CAD build for the part. Positions are in the model's coordinates, mm. A direction names the side the tool comes from. Give positions to 0.01 mm unless a question says otherwise; leave off trailing zeros. Order: outer loops, then holes, each group sorted by start corner. A loop starts at its lowest first (then second) coordinate and runs counter-clockwise, first axis right, second up.
Item 1: Band-saw the part on C-C on x = 0. Give the cut face in (y, z), plus the area to 3 significant figures.
Item 2: Band-saw the part on D-D on z = 9.25. Count the separate pieces of the cut face and the enclosed holes in it, plus the area to 3 significant figures.
Item 3: Band-saw the part on A-A on z = 1.25. Give the cut face in (x, y) (3 decimals), plus the area to 3 significant figures.
Item 4: Band-saw the part on B-B on x = 40. Give the cut face in (y, z), plus the area to 3 significant figures.
Item 5: Which spindle directions (+Z, -Z, +X, -X, +Y, -Y) get a long thin tool onto all of the face, cutting with end or side? Do faces 1 (the flat face through (25, 0, 0)), 2 (the flat face through (37.51, -14.46, 8.03)). Say none if no direction does.
Item 6: Wall check: L1, parallel to Y at x = 40, z = 2.5; L2, parallel to X at y = -1.5, z = 1.25; L3, parallel to Z at x = 6, y = -5. Give the ranges that are in metal, low to high.
Item 7: Two-plate mould, pull along X, no slides. Class faces 3 (the cylindrical face through (57.494, -0.447, 4.93)), 4 (the flat face through (16.612, -12.035, 3.819)), 5 (the flat face through (40, 15.5, 8)): released by +X, released by -X, zero draft, split by the parting line, or undercut.
Item 8: Flat gauge pins, fed straight in: P1, Ø5, axis at x = 28.5, z = 8.5, coming from the +Y side; P2, Ø1.4, axis at y = -12, z = 8, coming from the +X side; P3, Ø1.4, axis at x = 27.5, z = 7.5, coming from the -Y side; P4, Ø5.5, axis at x = 40, y = 0, coming from the -Z side. Where does each tip first touch, or does it go through?
```python
from build123d import *

# Parameters (mm, degrees)
SKETCH1_R           = 17.5
SKETCH1_R_2         = 10
SKETCH1_R_3         = 6
SKETCH1_R_4         = 3.5
SKETCH1_R_5         = 7.5
SKETCH1_R_6         = 5
SKETCH1_R_7         = 2
BOSS_EXTRUDE1_DEPTH = 10
SKETCH4_R           = 2
CUT_EXTRUDE2_DEPTH  = 11
CUT_EXTRUDE3_DEPTH  = 4
SKETCH5_R           = 2
CUT_EXTRUDE4_DEPTH  = 3
SKETCH6_R           = 5
CUT_EXTRUDE5_DEPTH  = 4
SKETCH7_R           = 6.5
CUT_EXTRUDE6_DEPTH  = 5


with BuildPart() as part:
    # Sketch1 → Boss-Extrude1 (new body)
    with BuildSketch(Plane.XY):
        with BuildLine():
            Line((35.625, 16.94430214), (-1.875, 7.261843774))
            ThreePointArc((-1.875, 7.261843774), (4.592793268, 5.929270613), (7.5, 0))
            ThreePointArc((7.5, 0), (4.592793268, -5.929270613), (-1.875, -7.261843774))
            Line((-1.875, -7.261843774), (35.625, -16.94430214))
            ThreePointArc((35.625, -16.94430214), (22.5, 0), (35.625, 16.94430214))
        make_face()
        with Locations((40, 0)):
            Circle(SKETCH1_R)
        with Locations((40, 0)):
            Circle(SKETCH1_R_2, mode=Mode.SUBTRACT)
        with Locations((40, 0)):
            Circle(SKETCH1_R_2)
        with Locations((40, 0)):
            Circle(SKETCH1_R_3, mode=Mode.SUBTRACT)
        with Locations((40, 0)):
            Circle(SKETCH1_R_3)
        with Locations((40, 0)):
            Circle(SKETCH1_R_4, mode=Mode.SUBTRACT)
        Circle(SKETCH1_R_5)
        Circle(SKETCH1_R_6, mode=Mode.SUBTRACT)
        Circle(SKETCH1_R_6)
        Circle(SKETCH1_R_7, mode=Mode.SUBTRACT)
    extrude(amount=BOSS_EXTRUDE1_DEPTH)

    # Sketch4 → Cut-Extrude2 (cut, through all)
    with BuildSketch(Plane.XY.offset(10)):
        with Locations((28, 0)):
            Circle(SKETCH4_R)
        with Locations((40, -12)):
            Circle(SKETCH4_R)
        with Locations((52, 0)):
            Circle(SKETCH4_R)
        with Locations((40, 12)):
            Circle(SKETCH4_R)
    extrude(amount=-CUT_EXTRUDE2_DEPTH, mode=Mode.SUBTRACT)

    # Sketch4_3 → Cut-Extrude3 (cut)
    with BuildSketch(Plane.XY.offset(10)):
        Polygon((38.550252532, 8.5), (41.449747468, 8.5), (43.5, 10.550252532), (43.5, 13.449747468), (41.449747468, 15.5), (38.550252532, 15.5), (36.5, 13.449747468), (36.5, 10.550252532), align=None)
        Polygon((50.550252532, 3.5), (48.5, 1.449747468), (48.5, -1.449747468), (50.550252532, -3.5), (53.449747468, -3.5), (55.5, -1.449747468), (55.5, 1.449747468), (53.449747468, 3.5), align=None)
        Polygon((43.5, -10.550252532), (41.449747468, -8.5), (38.550252532, -8.5), (36.5, -10.550252532), (36.5, -13.449747468), (38.550252532, -15.5), (41.449747468, -15.5), (43.5, -13.449747468), align=None)
        Polygon((29.449747468, -3.5), (31.5, -1.449747468), (31.5, 1.449747468), (29.449747468, 3.5), (26.550252532, 3.5), (24.5, 1.449747468), (24.5, -1.449747468), (26.550252532, -3.5), align=None)
    extrude(amount=-CUT_EXTRUDE3_DEPTH, mode=Mode.SUBTRACT)

    # Sketch5 → Cut-Extrude4 (cut)
    with BuildSketch(Plane.XY.offset(10)):
        with BuildLine():
            ThreePointArc((7.5, 0), (4.592793268, 5.929270613), (-1.875, 7.261843774))
            ThreePointArc((-1.875, 7.261843774), (-7.5, 0), (-1.875, -7.261843774))
            ThreePointArc((-1.875, -7.261843774), (4.592793268, -5.929270613), (7.5, 0))
        make_face()
        Circle(SKETCH5_R, mode=Mode.SUBTRACT)
        with BuildLine():
            Line((1.997983346, -8.261843774), (18.124999918, -12.425821548))
            ThreePointArc((18.124999918, -12.425821548), (11.187692481, -7.858779558), (8.5, 0))
            ThreePointArc((8.5, 0), (6.67955307, -5.256764288), (1.997983346, -8.261843774))
        make_face()
        with BuildLine():
            ThreePointArc((8.5, 0), (11.187692462, 7.858779534), (18.124999859, 12.425821533))
            Line((18.124999859, 12.425821533), (1.997983346, 8.261843774))
            ThreePointArc((1.997983346, 8.261843774), (6.67955307, 5.256764288), (8.5, 0))
        make_face()
        with BuildLine():
            ThreePointArc((1.997983346, -8.261843774), (6.67955307, -5.256764288), (8.5, 0))
            ThreePointArc((8.5, 0), (6.67955307, 5.256764288), (1.997983346, 8.261843774))
            Line((1.997983346, 8.261843774), (-1.875, 7.261843774))
            ThreePointArc((-1.875, 7.261843774), (4.592793268, 5.929270613), (7.5, 0))
            ThreePointArc((7.5, 0), (4.592793268, -5.929270613), (-1.875, -7.261843774))
            Line((-1.875, -7.261843774), (1.997983346, -8.261843774))
        make_face()
        with BuildLine():
            Line((-1.875, 7.261843774), (1.997983346, 8.261843774))
            ThreePointArc((1.997983346, 8.261843774), (-8.5, 0), (1.997983346, -8.261843774))
            Line((1.997983346, -8.261843774), (-1.875, -7.261843774))
            ThreePointArc((-1.875, -7.261843774), (-7.5, 0), (-1.875, 7.261843774))
        make_face()
    extrude(amount=-CUT_EXTRUDE4_DEPTH, mode=Mode.SUBTRACT)

    # Sketch6 → Cut-Extrude5 (cut)
    with BuildSketch(Plane.XY.offset(7)):
        Circle(SKETCH6_R)
    extrude(amount=-CUT_EXTRUDE5_DEPTH, mode=Mode.SUBTRACT)

    # Sketch7 → Cut-Extrude6 (cut)
    with BuildSketch(Plane(origin=(0, 0, 0), x_dir=(-1, 0, 0), z_dir=(0, 0, -1))):
        with Locations((-40, 0)):
            Circle(SKETCH7_R)
    extrude(amount=-CUT_EXTRUDE6_DEPTH, mode=Mode.SUBTRACT)


solid = part.part
```
The answers:
1. outline: (-7.75, 0) - (-2, 0) - (-2, 3) - (-5, 3) - (-5, 7) - (-7.75, 7) - close; (2, 0) - (7.75, 0) - (7.75, 7) - (5, 7) - (5, 3) - (2, 3) - close
1. area: 56.4 mm2
2. separate pieces: 1
2. enclosed holes: 5
2. area: 1,120 mm2
3. outline: (-1.875, -7.262) - (35.625, -16.944) arc R17.5 ccw (long way) to (35.625, 16.944) - (-1.875, 7.262) arc R7.5 ccw to start; hole circle Ø4 at (0, 0); hole circle Ø4 at (28, 0); hole circle Ø13 at (40, 0); hole circle Ø4 at (40, -12); hole circle Ø4 at (40, 12); hole circle Ø4 at (52, 0)
3. area: 1,410 mm2
4. outline: (-17.5, 0) - (-14, 0) - (-14, 6) - (-15.5, 6) - (-15.5, 10) - (-17.5, 10) - close; (-10, 0) - (-6.5, 0) - (-6.5, 5) - (-3.5, 5) - (-3.5, 10) - (-8.5, 10) - (-8.5, 6) - (-10, 6) - close; (3.5, 5) - (6.5, 5) - (6.5, 0) - (10, 0) - (10, 6) - (8.5, 6) - (8.5, 10) - (3.5, 10) - close; (14, 0) - (17.5, 0) - (17.5, 10) - (15.5, 10) - (15.5, 6) - (14, 6) - close
4. area: 146 mm2
5. face 1: -Z, +X, -X, +Y, -Y
5. face 2: +Z
6. L1: y = -17.5 to -14, -10 to -6.5, 6.5 to 10, 14 to 17.5
6. L2: x = -7.35 to -1.32, 1.32 to 26.68, 29.32 to 33.68, 46.32 to 50.68, 53.32 to 57.44
6. L3: z = 0 to 7
7. face 3: split by the parting line
7. face 4: released by -X
7. face 5: undercut
8. P1: stops at y = 15.75
8. P2: stops at x = 53.36
8. P3: stops at y = -15.03
8. P4: passes through
